Could you check a few things on this model? Use its own coordinates, in mm. Face numbers are marked on the shaded views. A direction names the side the tool comes from. Coordinates: 2 decimals unless noted, no trailing zeros. Order: outer loops, then holes, each group sorted by start corner. A loop starts at its lowest first (then second) coordinate and runs counter-clockwise, first axis right, second up. Notation, with made-up numbers: M 43,-21 L 93,-21 A17 ccw 93,-17 Z; hole C 20.5,43.25 d3. An arc over 180 degrees is marked long. One line per question, with ' | ' between items. Start each with the question number.
from build123d import *

# Parameters (mm, degrees)
F0_W      = 100.33
F0_H      = 137.16
F0_W_2    = 330.2
F0_H_2    = 304.8
F1_DEPTH  = 254
F2_W      = 50.8
F2_H      = 177.8
F3_DEPTH  = 25.4
F4_W      = 50.8
F4_H      = 177.8
F5_DEPTH  = 177.8
F6_W      = 63.5
F6_H      = 177.8
F7_DEPTH  = 25.4
F8_W      = 63.5
F8_H      = 177.8
F9_DEPTH  = 25.4
F10_W     = 88.9
F10_H     = 177.8
F11_DEPTH = 25.4
F12_R     = 6.35
F13_DEPTH = 228.6


with BuildPart() as f1:
    # F0 (on Top) → F1 (new body)
    with BuildSketch(Plane.XY):
        Polygon((847.09, 19.05), (-19.05, 19.05), (-19.05, -323.85), (-19.05, -850.9), (203.2, -850.9), (203.2, -647.7), (847.09, -647.7), align=None)
        with Locations((133.985, -577.85)):
            Rectangle(F0_W, F0_H, mode=Mode.SUBTRACT)
        Polygon((828.04, -628.65), (203.2, -628.65), (203.2, -501.65), (76.2, -501.65), (76.2, -654.05), (184.15, -654.05), (184.15, -831.85), (0, -831.85), (0, -323.85), (337.82, -323.85), (337.82, -292.1), (490.22, -292.1), (490.22, -323.85), (668.02, -323.85), (675.64, -323.85), (828.04, -323.85), (828.04, -450.85), (828.04, -458.47), align=None, mode=Mode.SUBTRACT)
        with Locations((165.1, -152.4)):
            Rectangle(F0_W_2, F0_H_2, mode=Mode.SUBTRACT)
        Polygon((337.82, -285.75), (337.82, -209.55), (420.37, -209.55), (420.37, -133.35), (490.22, -133.35), (490.22, -285.75), align=None, mode=Mode.SUBTRACT)
        Polygon((337.82, -203.2), (337.82, 0), (490.22, 0), (490.22, -127), (414.02, -127), (414.02, -203.2), align=None, mode=Mode.SUBTRACT)
        with Locations((662.94, -152.4)):
            Rectangle(F0_W_2, F0_H_2, mode=Mode.SUBTRACT)
    extrude(amount=F1_DEPTH)

    # F2 (on face) → F3 (cut)
    with BuildSketch(Plane.XZ.offset(292.1)):
        with Locations((452.12, 88.9)):
            Rectangle(F2_W, F2_H)
    extrude(amount=-F3_DEPTH, mode=Mode.SUBTRACT)

    # F4 (on face) → F5 (cut)
    with BuildSketch(Plane.YZ.offset(497.84)):
        with Locations((-88.9, 88.9)):
            Rectangle(F4_W, F4_H)
    extrude(amount=-F5_DEPTH, mode=Mode.SUBTRACT)

    # F6 (on face) → F7 (cut)
    with BuildSketch(Plane.XZ.offset(323.85)):
        with Locations((44.45, 88.9)):
            Rectangle(F6_W, F6_H)
    extrude(amount=-F7_DEPTH, mode=Mode.SUBTRACT)

    # F8 (on face) → F9 (cut)
    with BuildSketch(Plane.XZ.offset(323.85)):
        with Locations((542.29, 88.9)):
            Rectangle(F8_W, F8_H)
    extrude(amount=-F9_DEPTH, mode=Mode.SUBTRACT)

    # F10 (on face) → F11 (cut)
    with BuildSketch(Plane.XZ.offset(647.7)):
        with Locations((770.89, 88.9)):
            Rectangle(F10_W, F10_H)
    extrude(amount=-F11_DEPTH, mode=Mode.SUBTRACT)

    # F12 (on face) → F13 (cut)
    with BuildSketch(Plane.XZ.offset(209.55)):
        with Locations((361.95, 228.6)):
            Circle(F12_R)
    extrude(amount=-F13_DEPTH, mode=Mode.SUBTRACT)


solid = f1.part
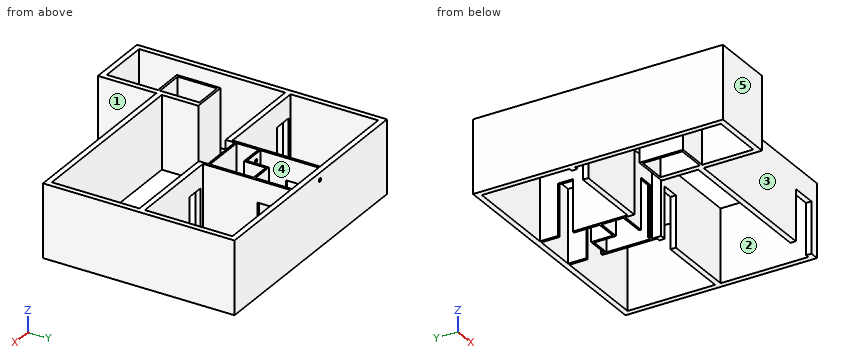
(1) On a 3-axis mill with a long thin cutter (end or side, diameter ignored), from which of +Z, -Z, +X, -X, +Y, -Y can I reach the whole of each face in a straight line? I mean the marked faces 4 and 5. Say none if no direction works.
(2) For P1, Ø4, axis at x = 333, z = 65.5, coming from the -Y side; P2, Ø4, axis at x = 495, y = -77.5, coming from the -Z side, each with a flat end and sliding along its axis, tell me the tip position at first contact or that it passes through.
(3) Imagine slicing it at C-C, the plane x = 154. Write out the boundary of the cut face in (y, z), plus the area to 3 significant figures.
(4) Imagine slicing it at D-D, the plane z = 159. Count the separate pieces of the cut face and the enclosed holes in it, plus the area to 3 significant figures.
(5) Imagine slicing it at B-B, the plane x = 397.5. Write out the boundary of the cut face in (y, z), plus the area to 3 significant figures.
(6) Imagine slicing it at A-A, the plane x = 786. Write out the boundary of the cut face in (y, z), plus the area to 3 significant figures.
(7) If I drill on line 1 along Y through (x, z) = (322.5, 223); line 2 along X through (y, z) = (-196, 21); line 3 along X through (y, z) = (-300, 72.5), over which ranges is the centre line in solid material (lowest first)? Write a range as from..to.
(8) We'd pull the mould along Y, two halves only. Please class the marked faces 1, 2 and 3: +Y half, -Y half, draft (parallel to the pull), parting line (faces both ways), or undercut.
Answers:
1) face 4: +Z, -Z | face 5: +Z, -Z, +X, -X, -Y
2) P1: y = -647.7 | P2: z = 177.8
3) outline: M -850.9,0 L -831.85,0 L -831.85,254 L -850.9,254 Z; M -654.05,0 L -646.43,0 L -646.43,254 L -654.05,254 Z; M -509.27,0 L -501.65,0 L -501.65,254 L -509.27,254 Z; M -323.85,0 L -304.8,0 L -304.8,254 L -323.85,254 Z; M 0,0 L 19.05,0 L 19.05,254 L 0,254 Z | area: 18,400 mm²
4) separate pieces: 2 | enclosed holes: 1 | area: 84,500 mm²
5) outline: M -647.7,0 L -628.65,0 L -628.65,254 L -647.7,254 Z; M -292.1,0 L -285.75,0 L -285.75,254 L -292.1,254 Z; M -209.55,0 L -203.2,0 L -203.2,254 L -209.55,254 Z; M 0,0 L 19.05,0 L 19.05,254 L 0,254 Z | area: 12,900 mm²
6) outline: M -647.7,177.8 L -628.65,177.8 L -628.65,254 L -647.7,254 Z; M -323.85,0 L -304.8,0 L -304.8,254 L -323.85,254 Z; M 0,0 L 19.05,0 L 19.05,254 L 0,254 Z | area: 11,100 mm²
7) line 1: -647.7..-628.65, -323.85..-304.8, 0..19.05 | line 2: -19.05..0, 330.2..337.82, 414.02..420.37, 490.22..497.84, 828.04..847.09 | line 3: -19.05..0, 330.2..337.82, 490.22..497.84, 828.04..847.09
8) face 1: draft | face 2: undercut | face 3: -Y half
